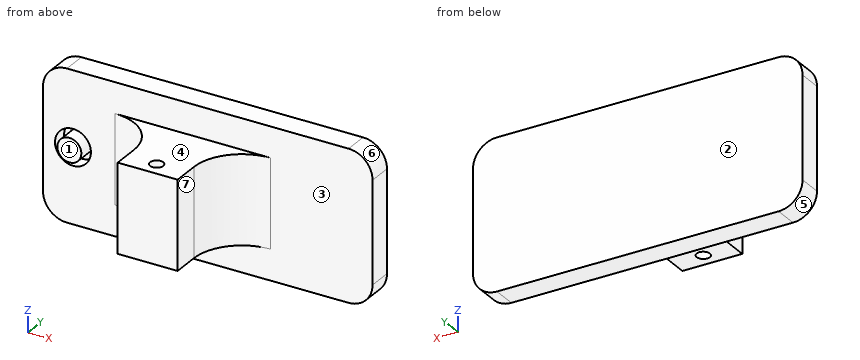
from build123d import *

# Parameters (mm, degrees)
SKETCH_1_W          = 55
SKETCH_1_H          = 25
EXTRUDE_1_DEPTH     = 4
SKETCH_2_R          = 3
CUT_EXTRUDE_1_DEPTH = 2.5
SKETCH_3_R          = 2
EXTRUDE_2_DEPTH     = 3.5
SKETCH_5_W          = 10
SKETCH_5_H          = 12.5
SKETCH_5_R          = 1.1
EXTRUDE_3_DEPTH     = 7.4
FILLET_1_R          = 8
FILLET_2_R          = 4


with BuildPart() as part:
    # 草图1 → 凸台-拉伸1 (new body)
    with BuildSketch(Plane(origin=(0, 0, 0), x_dir=(1, 0, 0), z_dir=(0, 1, 0))):
        Rectangle(SKETCH_1_W, SKETCH_1_H)
    extrude(amount=EXTRUDE_1_DEPTH)

    # 草图2 → 切除-拉伸1 (cut)
    with BuildSketch(Plane.XZ):
        with Locations(Location((-22.5, 0, 0), (0, 0, 270))):
            Circle(SKETCH_2_R)
    extrude(amount=-CUT_EXTRUDE_1_DEPTH, mode=Mode.SUBTRACT)

    # 草图3 → 凸台-拉伸2 (add)
    with BuildSketch(Plane.XZ.offset(-2.5)):
        with Locations(Location((-22.5, 0, 0), (0, 0, 270))):
            Circle(SKETCH_3_R)
    extrude(amount=EXTRUDE_2_DEPTH)

    # 草图5 → 凸台-拉伸3 (add, symmetric)
    with BuildSketch(Plane.XY):
        with Locations((-2.5, -6.25)):
            Rectangle(SKETCH_5_W, SKETCH_5_H)
        with Locations((-2.5, -10)):
            Circle(SKETCH_5_R, mode=Mode.SUBTRACT)
    extrude(amount=EXTRUDE_3_DEPTH, both=True)

    # 圆角1
    fillet_1_edges = [part.edges().sort_by_distance(p)[0] for p in [
        (2.5, 0, 0),
        (-7.5, 0, 0),
    ]]
    fillet(fillet_1_edges, radius=FILLET_1_R)

    # 圆角2
    fillet_2_edges = [part.edges().sort_by_distance(p)[0] for p in [
        (-27.5, 2, -12.5),
        (27.5, 2, -12.5),
        (27.5, 2, 12.5),
        (-27.5, 2, 12.5),
    ]]
    fillet(fillet_2_edges, radius=FILLET_2_R)


solid = part.part
Geometry: final body of the model. Coordinates: model frame, mm. Face numbers are marked on the shaded views. A direction names the side the tool comes from. Give positions to 0.01 mm unless a question says otherwise; leave off trailing zeros. Order: outer loops, then holes, each group sorted by start corner. A loop starts at its lowest first (then second) coordinate and runs counter-clockwise, first axis right, second up. Notation, with made-up numbers: (-26, 53.25) -> (13, 53.25) arc R24 ccw to (13, 67.25) -> close; hole circle Ø7 at (62, -23.5). An arc over 180 degrees is marked (long way). Answer as a JSON object with one key per item and string values.
Q1. First-contact query: pin 1 (1.2 mm diameter, centred on x = -23.5, z = -0.5, fed in from -Y); pin 2 (12.5 mm diameter, centred on x = 9.5, z = -2, fed in from -Y); pin 3 (2 mm diameter, centred on x = 2, y = -7.5, fed in from -Z); pin 4 (8 mm diameter, centred on x = -11, y = -3, fed in from +Z). Flat tips, straight axial feed; report the tip coordinate or a pass-through.
Entries:
{"pin 1": "stops at y = -1", "pin 2": "stops at y = -4.62", "pin 3": "stops at z = -7.4", "pin 4": "stops at z = 12.5"}
Q2. Material intervals for probe 1 along X at (y, z) = (1.5, 0); probe 2 along X at (y, z) = (0.5, 0.75); probe 3 along Z at (x, y) = (-21, 0.25), sorted ascending.
Entries:
{"probe 1": "x = -27.5 to -25.5, -24.5 to -20.5, -19.5 to 27.5", "probe 2": "x = -27.5 to -25.4, -24.35 to -20.65, -19.6 to 27.5", "probe 3": "z = -12.5 to -2.6, -1.32 to 1.32, 2.6 to 12.5"}
Q3. Section C-C (x = -2.5). Output: boundary loops of the cut face in (y, z), plus the area to 3 significant figures.
Entries:
{"outline": "(-12.5, -7.4) -> (-11.1, -7.4) -> (-11.1, 7.4) -> (-12.5, 7.4) -> close; (-8.9, -7.4) -> (0, -7.4) -> (0, -12.5) -> (4, -12.5) -> (4, 12.5) -> (0, 12.5) -> (0, 7.4) -> (-8.9, 7.4) -> close", "area": "252 mm^2"}
Q4. Section B-B (z = 0). Output: boundary loops of the cut face in (x, y), plus the area to 3 significant figures.
Entries:
{"outline": "(-27.5, 0) -> (-25.5, 0) -> (-25.5, 2.5) -> (-24.5, 2.5) -> (-24.5, -1) -> (-20.5, -1) -> (-20.5, 2.5) -> (-19.5, 2.5) -> (-19.5, 0) -> (-15.5, 0) arc R8 cw to (-7.5, -8) -> (-7.5, -12.5) -> (2.5, -12.5) -> (2.5, -8) arc R8 cw to (10.5, 0) -> (27.5, 0) -> (27.5, 4) -> (-27.5, 4) -> close; hole circle Ø2.2 at (-2.5, -10)", "area": "368 mm^2"}
Q5. Access query for the marked faces 1, 2, 3 and 4. Directions: +Z, -Z, +X, -X, +Y, -Y. A direction counts if a zero-diameter tool reaches every point of the face in a straight line with its end or side. Return the directions, or none.
Entries:
{"face 1": "+Z, -Z, -X, -Y", "face 2": "+Z, -Z, +X, -X, +Y", "face 3": "-Y", "face 4": "+Z, +X, -X, -Y"}
Q6. Section D-D (x = 9.5). Output: boundary loops of the cut face in (y, z), plus the area to 3 significant figures.
Entries:
{"outline": "(-0.06, -7.4) -> (0, -7.4) -> (0, -12.5) -> (4, -12.5) -> (4, 12.5) -> (0, 12.5) -> (0, 7.4) -> (-0.06, 7.4) -> close", "area": "101 mm^2"}
Q7. Section A-A (y = -10). Output: boundary loops of the cut face in (x, z).
Entries:
{"outline": "(-7.5, -7.4) -> (-3.6, -7.4) -> (-3.6, 7.4) -> (-7.5, 7.4) -> close; (-1.4, -7.4) -> (2.5, -7.4) -> (2.5, 7.4) -> (-1.4, 7.4) -> close"}
Q8. Draft query along Z for the marked faces 5, 6 and 7. Return one class per face: released by +Z, released by -Z, zero draft, split by the parting line, or undercut.
Entries:
{"face 5": "released by -Z", "face 6": "released by +Z", "face 7": "zero draft"}
